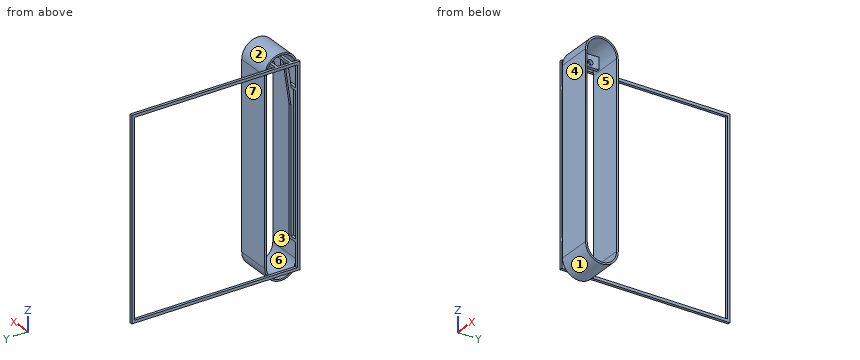
```python
from build123d import *

# Parameters (mm, degrees)
SKETCH1_W           = 1118.25
SKETCH1_H           = 944.035
BOSS_EXTRUDE1_DEPTH = 15.875
SKETCH2_W           = 15.875
SKETCH2_H           = 15.875
BOSS_EXTRUDE2_DEPTH = 55.785
SKETCH3_W           = 15.875
SKETCH3_H           = 15.875
BOSS_EXTRUDE3_DEPTH = 850
EXTRUDE_THIN2_START = 21
SKETCH4_W           = 850
SKETCH4_H           = 10
EXTRUDE_THIN2_DEPTH = 200
SKETCH5_W           = 15.875
SKETCH5_H           = 100
BOSS_EXTRUDE4_DEPTH = 120
SKETCH7_W           = 54
SKETCH7_H           = 100
SKETCH7_R           = 15
BOSS_EXTRUDE5_DEPTH = 20
BOSS_EXTRUDE6_DEPTH = 15.875
SKETCH11_W          = 100
SKETCH11_H          = 68.25
CUT_EXTRUDE1_DEPTH  = 20


with BuildPart() as part:
    # Sketch1 → Boss-Extrude1 (new body)
    with BuildSketch(Plane(origin=(0, 0, 0), x_dir=(0, 0, -1), z_dir=(1, 0, 0))):
        Polygon((-575, -487.8925), (-575, 487.8925), (575, 487.8925), (575, -487.8925), (559.125, -487.8925), (-559.125, -487.8925), align=None)
        Rectangle(SKETCH1_W, SKETCH1_H, mode=Mode.SUBTRACT)
    extrude(amount=BOSS_EXTRUDE1_DEPTH)

    # Sketch2 → Boss-Extrude2 (add)
    with BuildSketch(Plane(origin=(15.875, 0, 0), x_dir=(0, 0, -1), z_dir=(1, 0, 0))):
        with Locations((-417.0625, -479.955)):
            Rectangle(SKETCH2_W, SKETCH2_H)
        with Locations((417.0625, -479.955)):
            Rectangle(SKETCH2_W, SKETCH2_H)
    extrude(amount=BOSS_EXTRUDE2_DEPTH)

    # Sketch3 → Boss-Extrude3 (add)
    with BuildSketch(Plane.XY.offset(425)):
        with Locations((63.8125, -479.955)):
            Rectangle(SKETCH3_W, SKETCH3_H)
    extrude(amount=-BOSS_EXTRUDE3_DEPTH)

    # Sketch4 → Extrude-Thin2 (add)
    with BuildSketch(Plane(origin=(15.875, 0, 0), x_dir=(0, 0, -1), z_dir=(1, 0, 0)).offset(EXTRUDE_THIN2_START)):
        with Locations((0, -492.8925)):
            Rectangle(SKETCH4_W, SKETCH4_H)
        with BuildLine():
            Line((531.125, -497.8925), (-531.125, -497.8925))
            ThreePointArc((-531.125, -497.8925), (-626.125, -402.8925), (-531.125, -307.8925))
            Line((-531.125, -307.8925), (531.125, -307.8925))
            ThreePointArc((531.125, -307.8925), (626.125, -402.8925), (531.125, -497.8925))
        make_face()
        with BuildLine():
            Line((531.125, -487.8925), (-531.125, -487.8925))
            ThreePointArc((-531.125, -487.8925), (-616.125, -402.8925), (-531.125, -317.8925))
            Line((-531.125, -317.8925), (531.125, -317.8925))
            ThreePointArc((531.125, -317.8925), (616.125, -402.8925), (531.125, -487.8925))
        make_face(mode=Mode.SUBTRACT)
    extrude(amount=EXTRUDE_THIN2_DEPTH)

    # Sketch5 → Boss-Extrude4 (add)
    with BuildSketch(Plane(origin=(15.875, 0, 0), x_dir=(0, 0, -1), z_dir=(1, 0, 0))):
        with Locations((-567.0625, -402.8925)):
            Rectangle(SKETCH5_W, SKETCH5_H)
    extrude(amount=BOSS_EXTRUDE4_DEPTH)

    # Sketch7 → Boss-Extrude5 (add)
    with BuildSketch(Plane(origin=(135.875, 0, 0), x_dir=(0, 0, -1), z_dir=(1, 0, 0))):
        with Locations((-532.125, -402.8925)):
            Rectangle(SKETCH7_W, SKETCH7_H)
        with Locations((-531.125, -402.8925)):
            Circle(SKETCH7_R, mode=Mode.SUBTRACT)
    extrude(amount=-BOSS_EXTRUDE5_DEPTH)

    # Sketch9 → Boss-Extrude6 (add)
    with BuildSketch(Plane(origin=(71.75, 0, 0), x_dir=(0, 0, -1), z_dir=(1, 0, 0))):
        Polygon((-425, -472.0175), (-312.541363962, -472.0175), (-559.125, -436.856925616), (-559.125, -452.8925), align=None)
    extrude(amount=-BOSS_EXTRUDE6_DEPTH)

    # Sketch11 → Cut-Extrude1 (cut)
    with BuildSketch(Plane(origin=(0, 0, 559.125), x_dir=(-1, 0, 0), z_dir=(0, 0, -1))):
        with Locations((-65.875, -402.8925)):
            Rectangle(SKETCH11_W, SKETCH11_H)
    extrude(amount=-CUT_EXTRUDE1_DEPTH, mode=Mode.SUBTRACT)


solid = part.part
```
Read the model definition and answer for the solid it produces. Units are mm, in the model's axes. Face numbers are marked on the shaded views. A direction names the side the tool comes from. Round coordinates to 2 decimals unless told otherwise and drop trailing zeros. Loops run counter-clockwise (first coordinate to the right, second up) from the corner with the lowest first, then second, coordinate; pieces in that order, holes last. Notation, with made-up numbers: (-4.75, 18.5) -> (26.25, 18.5) arc R20 ccw to (26.25, 37.5) -> close; hole circle Ø5 at (42, -8). An arc over 180 degrees is marked (long way). One line per item, written item: value.
1) A cutting plane is placed at D-D (z = 381.5). Give the number of separate pieces and of enclosed holes in the cut face, and give its area (3 significant figures).
Answer list:
separate pieces: 4
enclosed holes: 0
area: 4,910 mm²
2) A cutting plane is placed at A-A (x = 97). Determine the outline of the cut face in (y, z) (1 decimal).
Answer list:
outline: (-497.9, -531.1) arc R95 ccw to (-307.9, -531.1) -> (-307.9, 531.1) arc R95 ccw to (-497.9, 531.1) -> close; (-452.9, 559.1) -> (-437, 559.1) -> (-437, 575) -> (-452.9, 575) -> close; (-368.8, 559.1) -> (-352.9, 559.1) -> (-352.9, 575) -> (-368.8, 575) -> close; hole (-487.9, -531.1) arc R85 ccw to (-317.9, -531.1) -> (-317.9, 531.1) arc R85 ccw to (-487.9, 531.1) -> close
3) For the marked faces 5, 6 and 7, determine the directions among +Z, -Z, +X, -X, +Y, -Y from which every point of the face is accessible in a straight line to the end or side of a thin tool.
Answer list:
face 5: +X, -X
face 6: +X
face 7: +Z, -Z, +X, -X, +Y
4) A cutting plane is placed at B-B (x = 188). Determine the outline of the cut face in (y, z) (1 decimal).
Answer list:
outline: (-497.9, -531.1) arc R95 ccw to (-307.9, -531.1) -> (-307.9, 531.1) arc R95 ccw to (-497.9, 531.1) -> close; hole (-487.9, -531.1) arc R85 ccw to (-317.9, -531.1) -> (-317.9, 531.1) arc R85 ccw to (-487.9, 531.1) -> close
5) A cutting plane is placed at C-C (y = -130). Determine the outline of the cut face in (x, z) (3 decimals).
Answer list:
outline: (0, -575) -> (15.875, -575) -> (15.875, -559.125) -> (0, -559.125) -> close; (0, 559.125) -> (15.875, 559.125) -> (15.875, 575) -> (0, 575) -> close
6) Flat-ended cylindrical pins translate along their axes: P1, Ø12.5, axis at x = 55.5, y = -476.5, coming from the +Z side; P2, Ø5, axis at y = -480.5, z = 169.5, coming from the +X side; P3, Ø1.5, axis at x = 137, z = 200, coming from the +Y side. Find the tip coordinate at first contact, or state that the pin passes through.
Answer list:
P1: stops at z = 598.12
P2: stops at x = 71.75
P3: stops at y = -307.89
7) The mould has two halves that part along Z. Classify the marked faces 1, 2, 3 and 4: pulls with the +Z half, pulls with the -Z half, needs draft (parallel to the pull), parting line crosses it, or undercut.
Answer list:
face 1: pulls with the -Z half
face 2: pulls with the +Z half
face 3: undercut
face 4: needs draft
8) Consider L1, parallel to Y at x = 169.5, z = 118; L2, parallel to Y at x = 59.5, z = 119.5; L3, parallel to Z at x = 10, y = 211.5 (3 decimals). Determine where each line is inside the solid, lowest interval first. Write a range as [from, to].
Answer list:
L1: y = [-497.89, -487.89], [-317.89, -307.89]
L2: y = [-497.89, -472.02], [-317.89, -307.89]
L3: z = [-575, -559.125], [559.125, 575]
